Read the model definition and answer for the solid it produces. Units are mm, in the model's axes. A direction names the side the tool comes from. Give positions to 0.01 mm unless a question says otherwise; leave off trailing zeros. Write each loop counter-clockwise with the first axis right and the second up, starting at its lowest first coordinate (ties: lowest second). Pieces come first, ordered by that corner, then holes. Notation, with made-up numbers: (14.5, 86.25) -> (68.5, 86.25) arc R34 cw to (68.5, 123.25) -> close; hole circle Ø1 at (21.25, 33.25). An arc over 180 degrees is marked (long way). Write item = value, one per line.
from build123d import *

# Parameters (mm, degrees)
SKETCH1_R                = 6
BOSS_EXTRUDE1_DEPTH      = 10
BOSS_EXTRUDE2_DEPTH      = 40
BOSS_EXTRUDE3_DEPTH      = 30
BOSS_EXTRUDE3_DEPTH_BACK = 50
SKETCH2_3_R              = 25
SKETCH3_R                = 17.5
BOSS_EXTRUDE4_DEPTH      = 16
SKETCH4_R                = 10
CUT_EXTRUDE1_DEPTH       = 143


with BuildPart() as part:
    # Sketch1 → Boss-Extrude1 (new body)
    with BuildSketch(Plane.XY):
        with BuildLine():
            Line((-77.756941547, 20), (-122.756941547, 20))
            ThreePointArc((-122.756941547, 20), (-125.674902222, 0), (-122.756941547, -20))
            Line((-122.756941547, -20), (-77.756941547, -20))
            Line((-77.756941547, -20), (-77.756941547, 20))
        make_face()
        with Locations((-102.756941547, 0)):
            Circle(SKETCH1_R, mode=Mode.SUBTRACT)
    boss_extrude1 = extrude(amount=BOSS_EXTRUDE1_DEPTH)

    # Sketch2 → Boss-Extrude2 (add)
    with BuildSketch(Plane(origin=(0, 20, 0), x_dir=(1, 0, 0), z_dir=(0, 1, 0))):
        with BuildLine():
            Line((-87.756941547, 0), (-77.756941547, 0))
            Line((-77.756941547, 0), (-77.756941547, 10))
            Line((-77.756941547, 10), (-12.756941547, 10))
            ThreePointArc((-12.756941547, 10), (-30.434611076, 17.32233047), (-37.756941547, 35))
            Line((-37.756941547, 35), (-47.756941547, 35))
            Line((-47.756941547, 35), (-47.756941547, 20))
            Line((-47.756941547, 20), (-87.756941547, 20))
            Line((-87.756941547, 20), (-87.756941547, 0))
        make_face()
    boss_extrude2 = extrude(amount=-BOSS_EXTRUDE2_DEPTH)

    # Sketch2<3> → Boss-Extrude3 (add, two sides: drawn at the far end of the back side and taken through both)
    with BuildSketch(Plane(origin=(0, 20, 0), x_dir=(1, 0, 0), z_dir=(0, 1, 0)).offset(-BOSS_EXTRUDE3_DEPTH_BACK)):
        with Locations(Location((-12.756941547, 35, 0), (0, 0, 270))):
            Circle(SKETCH2_3_R)
    extrude(amount=BOSS_EXTRUDE3_DEPTH + BOSS_EXTRUDE3_DEPTH_BACK)

    # Sketch3 → Boss-Extrude4 (add)
    with BuildSketch(Plane(origin=(0, 50, 0), x_dir=(1, 0, 0), z_dir=(0, 1, 0))):
        with Locations(Location((-12.756941547, 35, 0), (0, 0, 270))):
            Circle(SKETCH3_R)
    extrude(amount=BOSS_EXTRUDE4_DEPTH)

    # Sketch4 → Cut-Extrude1 (cut)
    with BuildSketch(Plane(origin=(0, 66, 0), x_dir=(1, 0, 0), z_dir=(0, 1, 0))):
        with Locations(Location((-12.756941547, 35, 0), (0, 0, 270))):
            Circle(SKETCH4_R)
    extrude(amount=-CUT_EXTRUDE1_DEPTH, mode=Mode.SUBTRACT)

    # Mirror11: Boss-Extrude2 across plane
    add(boss_extrude2.mirror(Plane(origin=(0, 0, -35), x_dir=(1, 0, 0), z_dir=(0, 0, -1))))

    # Mirror12: Boss-Extrude1 across plane
    add(boss_extrude1.mirror(Plane(origin=(0, 0, -35), x_dir=(1, 0, 0), z_dir=(0, 0, -1))))


solid = part.part
(1) Consider L1, parallel to Z at x = -70.5, y = 17.5; L2, parallel to Z at x = -12.5, y = 59.5; L3, parallel to Y at x = -50, z = -14.5. Determine where each line is inside the solid, lowest interval first.
Checks:
L1 = -60 to -50, -20 to -10
L2 = -52.5 to -45, -25 to -17.5
L3 = -20 to 20
(2) The part is cut by section D-D on x = -1. Determine the outline of the cut face in (y, z), plus the area to 3 significant figures.
Checks:
outline = (-30, -57.06) -> (50, -57.06) -> (50, -47.96) -> (66, -47.96) -> (66, -22.04) -> (50, -22.04) -> (50, -12.94) -> (-30, -12.94) -> close
area = 3,940 mm²
(3) For a pull along X with two mould halves and no side action, classify faces 1 (the cylindrical face through (-108.75, 0.26, 4.93)), 2 (the flat face through (-76, 20, -51)), 3 (the flat face through (-87.757, 0, -60)) as released by +X, released by -X, zero draft, split by the parting line, or undercut.
Checks:
face_1 = undercut
face_2 = zero draft
face_3 = released by -X
(4) A tool of negligible diameter and unlimited length cuts with its end or side. For faces 4 (the flat face through (-77.757, 0, -70)), 5 (the flat face through (-46, 0, -10)), 6 (the cylindrical face through (-7.5, 57.89, -18.31)), from which of +Z, -Z, +X, -X, +Y, -Y can it reach the whole face along a straight path? Write none if from no direction.
Checks:
face_4 = -Z, +X, +Y, -Y
face_5 = +Z, +X, +Y, -Y
face_6 = +Y
(5) The part is cut by section C-C on z = -35. Determine the outline of the cut face in (x, y).
Checks:
outline = (-47.76, -20) -> (-37.76, -20) -> (-37.76, -30) -> (-22.76, -30) -> (-22.76, 66) -> (-30.26, 66) -> (-30.26, 50) -> (-37.76, 50) -> (-37.76, 20) -> (-47.76, 20) -> close; (-2.76, -30) -> (12.24, -30) -> (12.24, 50) -> (4.74, 50) -> (4.74, 66) -> (-2.76, 66) -> close
(6) The part is cut by section B-B on x = -66.5. Determine the outline of the cut face in (y, z).
Checks:
outline = (-20, -60) -> (20, -60) -> (20, -50) -> (-20, -50) -> close; (-20, -20) -> (20, -20) -> (20, -10) -> (-20, -10) -> close
(7) The part is cut by section A-A on y = 0. Determine the outline of the cut face in (x, z), plus the area to 3 significant figures.
Checks:
outline = (-125.67, -80) -> (-108.76, -80) -> (-108.76, -70) -> (-125.67, -70) -> close; (-125.67, 0) -> (-108.76, 0) -> (-108.76, 10) -> (-125.67, 10) -> close; (-96.76, -80) -> (-77.76, -80) -> (-77.76, -60) -> (-12.76, -60) arc R25 ccw to (-12.76, -10) -> (-77.76, -10) -> (-77.76, 10) -> (-96.76, 10) -> (-96.76, 0) -> (-87.76, 0) -> (-87.76, -20) -> (-47.76, -20) -> (-47.76, -50) -> (-87.76, -50) -> (-87.76, -70) -> (-96.76, -70) -> close; hole circle Ø20 at (-12.76, -35)
area = 4,140 mm²
(8) Given P1, Ø1, axis at y = 12.5, z = -42, coming from the -X side; P2, Ø16, axis at y = -6.5, z = -72.5, coming from the +X side; P3, Ø8, axis at y = -15.5, z = -37.5, coming from the +X side, each flat-ended and moving along its own axis, determine where each tip first touches the part or whether it passes through.
Checks:
P1 = -47.76
P2 = -77.76
P3 = 12.24
